Could you check a few things on this model? Use its own coordinates, in mm. A direction names the side the tool comes from. Round coordinates to 2 decimals unless told otherwise and drop trailing zeros. Write each loop counter-clockwise with the first axis right and the second up, starting at its lowest first coordinate (ties: lowest second). Pieces come first, ordered by that corner, then holes. Notation, with made-up numbers: (-11, -23) -> (45, -23) arc R16 cw to (45, 3) -> close; hole circle Ø3 at (-10, 44). An arc over 180 degrees is marked (long way). Return JSON: item names as keys, results as strings.
from build123d import *

# Parameters (mm, degrees)
SKETCH1_R            = 7.6
BOSS_EXTRUDE1_DEPTH  = 25
SKETCH2_W            = 30
SKETCH2_H            = 27
BOSS_EXTRUDE2_DEPTH  = 25
SKETCH3_R            = 7.6
BOSS_EXTRUDE3_DEPTH  = 2
CHAMFER1_SIZE        = 5
SKETCH5_W            = 25
SKETCH5_H            = 4
BOSS_EXTRUDE4_DEPTH  = 15
SKETCH6_R            = 2.25
CUT_EXTRUDE2_DEPTH   = 15
FILLET1_R            = 10
FILLET1_OF_MIRROR2_R = 10
SKETCH7_R            = 2.25
CUT_EXTRUDE3_DEPTH   = 15
CUT_EXTRUDE4_DEPTH   = 15
SKETCH9_R            = 2.1
CUT_EXTRUDE5_DEPTH   = 28.468092804
CUT_EXTRUDE6_DEPTH   = 5


with BuildPart() as part:
    # Sketch1 → Boss-Extrude1 (new body)
    with BuildSketch(Plane.XY):
        with BuildLine():
            Line((-90, 0), (-90, 17))
            Line((-90, 17), (90, 17))
            Line((90, 17), (90, 0))
            ThreePointArc((90, 0), (80, -10), (70, 0))
            Line((70, 0), (70, 13))
            Line((70, 13), (-70, 13))
            Line((-70, 13), (-70, 0))
            ThreePointArc((-70, 0), (-80, -10), (-90, 0))
        make_face()
        with Locations((-80, 0)):
            Circle(SKETCH1_R, mode=Mode.SUBTRACT)
        with Locations((80, 0)):
            Circle(SKETCH1_R, mode=Mode.SUBTRACT)
    extrude(amount=BOSS_EXTRUDE1_DEPTH)

    # Sketch2 → Boss-Extrude2 (add)
    with BuildSketch(Plane(origin=(0, 0, 0), x_dir=(-1, 0, 0), z_dir=(0, 0, -1))):
        with Locations((-31, 3.5)):
            Rectangle(SKETCH2_W, SKETCH2_H)
    extrude(amount=-BOSS_EXTRUDE2_DEPTH)

    # Sketch3 → Boss-Extrude3 (add)
    with BuildSketch(Plane(origin=(0, 0, 0), x_dir=(-1, 0, 0), z_dir=(0, 0, -1))):
        with BuildLine():
            Line((80, -10), (-12, -10))
            Line((-12, -10), (-42, -10))
            Line((-42, -10), (-80, -10))
            ThreePointArc((-80, -10), (-87.071067812, -7.071067812), (-90, 0))
            Line((-90, 0), (-90, 17))
            Line((-90, 17), (90, 17))
            Line((90, 17), (90, 0))
            ThreePointArc((90, 0), (87.071067812, -7.071067812), (80, -10))
        make_face()
        with Locations((80, 0)):
            Circle(SKETCH3_R, mode=Mode.SUBTRACT)
        with Locations((-80, 0)):
            Circle(SKETCH3_R, mode=Mode.SUBTRACT)
    boss_extrude3 = extrude(amount=-BOSS_EXTRUDE3_DEPTH)

    # Mirror1: Boss-Extrude3 across plane
    add(boss_extrude3.mirror(Plane.XY.offset(12.5)))

    # Chamfer1
    chamfer1_edges = [part.edges().sort_by_distance(p)[0] for p in [
        (70, 13, 12.5),
        (-70, 13, 12.5),
    ]]
    chamfer(chamfer1_edges, length=CHAMFER1_SIZE)

    # Sketch5 → Boss-Extrude4 (add)
    with BuildSketch(Plane.ZY.offset(90)):
        with Locations((12.5, 15)):
            Rectangle(SKETCH5_W, SKETCH5_H)
    boss_extrude4 = extrude(amount=BOSS_EXTRUDE4_DEPTH)

    # Sketch6 → Cut-Extrude2 (cut)
    with BuildSketch(Plane(origin=(0, 13, 0), x_dir=(-1, 0, 0), z_dir=(0, -1, 0))):
        with Locations((97.5, -12.5)):
            Circle(SKETCH6_R)
    cut_extrude2 = extrude(amount=-CUT_EXTRUDE2_DEPTH, mode=Mode.SUBTRACT)

    # Fillet1
    fillet1_edges = [part.edges().sort_by_distance(p)[0] for p in [
        (-105, 15, 0),
        (-105, 15, 25),
    ]]
    fillet(fillet1_edges, radius=FILLET1_R)

    # Mirror2: Boss-Extrude4 across plane
    add(boss_extrude4.mirror(Plane(origin=(0, 0, 0), x_dir=(0, 0, 1), z_dir=(1, 0, 0))))

    # Fillet1 of Mirror2
    fillet1_of_mirror2_edges = [part.edges().sort_by_distance(p)[0] for p in [
        (105, 15, 0),
        (105, 15, 25),
    ]]
    fillet(fillet1_of_mirror2_edges, radius=FILLET1_OF_MIRROR2_R)

    # Mirror4: Cut-Extrude2 across plane
    add(cut_extrude2.mirror(Plane(origin=(0, 0, 0), x_dir=(0, 0, 1), z_dir=(1, 0, 0))), mode=Mode.SUBTRACT)

    # Sketch7 → Cut-Extrude3 (cut)
    with BuildSketch(Plane(origin=(0, 17, 0), x_dir=(1, 0, 0), z_dir=(0, 1, 0))):
        with Locations((-57.5, -12.5)):
            Circle(SKETCH7_R)
        with Locations((57.5, -12.5)):
            Circle(SKETCH7_R)
    extrude(amount=-CUT_EXTRUDE3_DEPTH, mode=Mode.SUBTRACT)

    # Sketch8 → Cut-Extrude4 (cut)
    with BuildSketch(Plane.XZ.offset(10)):
        with BuildLine():
            Line((21.95, 19), (20, 19))
            Line((20, 19), (20, 17.05))
            ThreePointArc((20, 17.05), (21.378858223, 17.621141777), (21.95, 19))
        make_face()
        with BuildLine():
            Line((20, 17.05), (20, 19))
            Line((20, 19), (21.95, 19))
            ThreePointArc((21.95, 19), (18.621141777, 20.378858223), (20, 17.05))
        make_face()
        with BuildLine():
            ThreePointArc((43.95, 19), (42, 20.95), (40.05, 19))
            Line((40.05, 19), (42, 19))
            Line((42, 19), (42, 17.05))
            ThreePointArc((42, 17.05), (43.378858223, 17.621141777), (43.95, 19))
        make_face()
        with BuildLine():
            Line((42, 19), (40.05, 19))
            ThreePointArc((40.05, 19), (40.621141777, 17.621141777), (42, 17.05))
            Line((42, 17.05), (42, 19))
        make_face()
        with BuildLine():
            ThreePointArc((42, 7.95), (40.621141777, 7.378858223), (40.05, 6))
            Line((40.05, 6), (42, 6))
            Line((42, 6), (42, 7.95))
        make_face()
        with BuildLine():
            Line((42, 6), (40.05, 6))
            ThreePointArc((40.05, 6), (42, 4.05), (43.95, 6))
            ThreePointArc((43.95, 6), (43.378858223, 7.378858223), (42, 7.95))
            Line((42, 7.95), (42, 6))
        make_face()
        with BuildLine():
            ThreePointArc((21.95, 6), (21.378858223, 7.378858223), (20, 7.95))
            Line((20, 7.95), (20, 6))
            Line((20, 6), (21.95, 6))
        make_face()
        with BuildLine():
            Line((20, 6), (20, 7.95))
            ThreePointArc((20, 7.95), (18.621141777, 4.621141777), (21.95, 6))
            Line((21.95, 6), (20, 6))
        make_face()
    extrude(amount=-CUT_EXTRUDE4_DEPTH, mode=Mode.SUBTRACT)

    # Sketch9 → Cut-Extrude5 (cut)
    with BuildSketch(Plane.XY.offset(25)):
        with Locations((31, -5)):
            Circle(SKETCH9_R)
    extrude(amount=-CUT_EXTRUDE5_DEPTH, mode=Mode.SUBTRACT)

    # Sketch10 → Cut-Extrude6 (cut)
    with BuildSketch(Plane(origin=(0, 0, 0), x_dir=(-1, 0, 0), z_dir=(0, 0, -1))):
        Polygon((-26.669872981, -5), (-28.834936491, -1.25), (-33.165063509, -1.25), (-35.330127019, -5), (-33.165063509, -8.75), (-28.834936491, -8.75), align=None)
    extrude(amount=-CUT_EXTRUDE6_DEPTH, mode=Mode.SUBTRACT)


solid = part.part
1) Will these pins go through, and if not, where does the flat tip stop? pin 1 Ø4 at (y, z) = (4, 10.5) entering from +X; pin 2 Ø3.5 at (x, z) = (97.5, 12.5) entering from +Y; pin 3 Ø1 at (y, z) = (8, 14) entering from -X; pin 4 Ø7.5 at (x, z) = (-95, 14) entering from -Y.
Return value:
{"pin 1": "x = 90", "pin 2": "through", "pin 3": "x = -90", "pin 4": "y = 13"}
2) I want a section at A-A, the plane x = 57.5. Please give me the cut outline in (y, z).
Return value:
{"outline": "(-10, 0) -> (17, 0) -> (17, 10.25) -> (13, 10.25) -> (13, 2) -> (-10, 2) -> close; (-10, 23) -> (13, 23) -> (13, 14.75) -> (17, 14.75) -> (17, 25) -> (-10, 25) -> close"}
3) Thinking about a two-plate mould opening in Y: for faces 4 (the face through (34.26, -6.85, 2.46)), 5 (the face through (-59.748, 15.028, 12.401)), 6 (the face through (-94, 13, 12)), which applies, pulls with the +Y half, pulls with the -Y half, needs draft (parallel to the pull), parting line crosses it, or undercut?
Return value:
{"face 4": "undercut", "face 5": "needs draft", "face 6": "pulls with the -Y half"}
4) I want a section at B-B, the plane x = 5.5. Please give me the cut outline in (y, z), and give its area (3 significant figures).
Return value:
{"outline": "(-10, 0) -> (17, 0) -> (17, 25) -> (-10, 25) -> (-10, 23) -> (13, 23) -> (13, 2) -> (-10, 2) -> close", "area": "192 mm²"}
5) If I drill on probe 1 along X at (y, z) = (15.15, 12.5); probe 2 along Z at (x, y) = (20, -6.5); probe 3 along Z at (x, y) = (-9.5, -1), over which ranges is the centre line in solid material (lowest first)? Write a range as [from, to].
Return value:
{"probe 1": "[-105, -99.75], [-95.25, -59.75], [-55.25, 55.25], [59.75, 95.25], [99.75, 105]", "probe 2": "[0, 4.05], [7.95, 17.05], [20.95, 25]", "probe 3": "[0, 2], [23, 25]"}
6) For faces 1 (the face through (31, -8.75, 2)), 2 (the face through (-68, 10, 12)), 3 (the face through (74.4, 5.14, 12.32)), which set-ups out of +Z, -Z, +X, -X, +Y, -Y let a thin tool reach every point of the face, with its end or its side?
Return value:
{"face 1": "-Z", "face 2": "-Y", "face 3": "+Z, -Z"}
